Verification items for the finished model (mm, model axes). A direction names the side the tool comes from. Give positions to 0.01 mm unless a question says otherwise; leave off trailing zeros. Order: outer loops, then holes, each group sorted by start corner. A loop starts at its lowest first (then second) coordinate and runs counter-clockwise, first axis right, second up.
(1) Sectioned sample at B-B on x = -2. Record the cut outline in (y, z) (3 decimals).
(2) Scan lines: L1, parallel to X at y = 78.5, z = 5.75 (3 decimals); L2, parallel to Y at x = 0, z = 7.5 (3 decimals); L3, parallel to X at y = 57, z = 9. Record each from-to range of solid material in increasing order.
(3) Gauge pin test, flat ends, axial feed: pin 1 (5 mm diameter, centred on x = -50, z = 6.5, fed in from -Y); pin 2 (4 mm diameter, centred on y = 75.5, z = 7.5, fed in from +X); pin 3 (6.5 mm diameter, centred on x = -14, z = 4.5, fed in from +Y) (3 decimals). Record the tip position at first contact, or that the pin passes through.
(4) Mould release check, pull along Y, two halves, no side actions. Record for faces 1 (the face through (-38.1, 73, 6)), 2 (the face through (98.28, 16.3, 6.26)), 3 (the face through (51, 60.325, 6)): pulls with the +Y half, pulls with the -Y half, needs draft (parallel to the pull), parting line crosses it, or undercut.
(5) Sectioned sample at A-A on y = 16. Record the cut outline in (x, z), plus the area to 3 significant figures.
(6) Sectioned sample at C-C on y = -18.5. Record the cut outline in (x, z), plus the area to 3 significant figures.
(7) Sectioned sample at D-D on y = 79. Record the cut outline in (x, z) (3 decimals), plus the area to 3 significant figures.
(8) Access from +Z, -Z, +X, -X, +Y, -Y to the whole of each face (thin tool, end or side, straight path). Record for faces 4 (the face through (-57, 92.075, 6)), 5 (the face through (1, 53.975, 6)), 6 (the face through (-51, 60.325, 6)).
```python
from build123d import *

# Parameters (mm, degrees)
F0_R     = 38.1
F0_R_2   = 22.225
F1_DEPTH = 12.7
F4_W     = 6.35
F4_H     = 25.4
F5_DEPTH = 12.7
F6_W     = 6.35
F6_H     = 25.4
F7_DEPTH = 12.7


with BuildPart() as f1:
    # F0 (on Top) → F1 (new body)
    with BuildSketch(Plane.XY):
        with BuildLine():
            Line((-76.2, 41.275), (-41.964057, -22.520182))
            ThreePointArc((-41.964057, -22.520182), (-14.468928, -45.373899), (21.180573, -42.655878))
            Line((21.180573, -42.655878), (82.558344, -12.179039))
            ThreePointArc((82.558344, -12.179039), (98.224966, 16.789683), (76.2, 41.275))
            Line((76.2, 41.275), (76.2, 92.075))
            Line((76.2, 92.075), (38.1, 92.075))
            Line((38.1, 92.075), (38.1, 53.975))
            Line((38.1, 53.975), (-38.1, 53.975))
            Line((-38.1, 53.975), (-38.1, 92.075))
            Line((-38.1, 92.075), (-76.2, 92.075))
            Line((-76.2, 92.075), (-76.2, 41.275))
        make_face()
        Circle(F0_R, mode=Mode.SUBTRACT)
        with Locations((69.85, 13.414488)):
            Circle(F0_R_2, mode=Mode.SUBTRACT)
    extrude(amount=F1_DEPTH)

    # F4 (on face) → F5 (cut, through all)
    with BuildSketch(Plane.XY.offset(12.7)):
        with Locations((-50.8, 73.025)):
            Rectangle(F4_W, F4_H)
    extrude(amount=-F5_DEPTH, mode=Mode.SUBTRACT)

    # F6 (on face) → F7 (cut, through all)
    with BuildSketch(Plane.XY.offset(12.7)):
        with Locations((50.8, 73.025)):
            Rectangle(F6_W, F6_H)
    extrude(amount=-F7_DEPTH, mode=Mode.SUBTRACT)


solid = f1.part
```
Ans:
1. outline: (-47.583, 0) - (-38.047, 0) - (-38.047, 12.7) - (-47.583, 12.7) - close; (38.047, 0) - (53.975, 0) - (53.975, 12.7) - (38.047, 12.7) - close
2. L1: x = -76.2 to -53.975, -47.625 to -38.1, 38.1 to 47.625, 53.975 to 76.2
2. L2: y = -47.625 to -38.1, 38.1 to 53.975
2. L3: x = -76.2 to -38.1, 38.1 to 76.2
3. pin 1: stops at y = -12.2
3. pin 2: stops at x = 76.2
3. pin 3: stops at y = 53.975
4. face 1: needs draft
4. face 2: parting line crosses it
4. face 3: undercut
5. outline: (-62.64, 0) - (-34.58, 0) - (-34.58, 12.7) - (-62.64, 12.7) - close; (34.58, 0) - (47.78, 0) - (47.78, 12.7) - (34.58, 12.7) - close; (91.92, 0) - (98.31, 0) - (98.31, 12.7) - (91.92, 12.7) - close
5. area: 605 mm2
6. outline: (-44.12, 0) - (-33.31, 0) - (-33.31, 12.7) - (-44.12, 12.7) - close; (33.31, 0) - (69.83, 0) - (69.83, 12.7) - (33.31, 12.7) - close
6. area: 601 mm2
7. outline: (-76.2, 0) - (-53.975, 0) - (-53.975, 12.7) - (-76.2, 12.7) - close; (-47.625, 0) - (-38.1, 0) - (-38.1, 12.7) - (-47.625, 12.7) - close; (38.1, 0) - (47.625, 0) - (47.625, 12.7) - (38.1, 12.7) - close; (53.975, 0) - (76.2, 0) - (76.2, 12.7) - (53.975, 12.7) - close
7. area: 806 mm2
8. face 4: +Z, -Z, +X, -X, +Y
8. face 5: +Z, -Z, +Y
8. face 6: +Z, -Z
